```python
from build123d import *

# Parameters (mm, degrees)
SKETCH2_R          = 25
SKETCH2_R_2        = 17.5
CUT_EXTRUDE1_DEPTH = 7
SKETCH3_R          = 3
CUT_EXTRUDE2_DEPTH = 25


with BuildPart() as part:
    # Sketch1 → Revolve1 (revolve)
    with BuildSketch(Plane.XY):
        Polygon((0, 20), (0, 4), (25, 4), (25, 25), (5, 25), (5, 20), align=None)
    revolve(axis=Axis((25, 0, 0), (-1, 0, 0)))

    # Mirror1: part across plane


with BuildPart() as part_1:
    add(part.part)
    add(part.part.mirror(Plane(origin=(0, 0, 0), x_dir=(0, 0, 1), z_dir=(1, 0, 0))))

    # Sketch2 → Cut-Extrude1 (cut)
    with BuildSketch(Plane.ZY.offset(25)):
        with Locations(Location((0, 0, 0), (0, 0, 90))):
            Circle(SKETCH2_R)
        with Locations(Location((0, 0, 0), (0, 0, 270))):
            Circle(SKETCH2_R_2, mode=Mode.SUBTRACT)
    extrude(amount=-CUT_EXTRUDE1_DEPTH, mode=Mode.SUBTRACT)

    # Sketch3 → Cut-Extrude2 (cut)
    with BuildSketch(Plane(origin=(0, 25, 0), x_dir=(1, 0, 0), z_dir=(0, 1, 0))):
        with Locations(Location((-11.5, 0, 0), (0, 0, 180))):
            Circle(SKETCH3_R)
    extrude(amount=-CUT_EXTRUDE2_DEPTH, mode=Mode.SUBTRACT)


solid = part_1.part
```
CAD build for the part. Positions are in the model's coordinates, mm. A direction names the side the tool comes from. Round coordinates to 2 decimals unless told otherwise and drop trailing zeros. Loops run counter-clockwise (first coordinate to the right, second up) from the corner with the lowest first, then second, coordinate; pieces in that order, holes last. Notation, with made-up numbers: (-38, 18.5) - (-10, 18.5) arc R17 cw to (-10, 40.5) - close; hole circle Ø8 at (11.25, 74.5). An arc over 180 degrees is marked (long way). Return JSON: item names as keys, results as strings. Group by question number.
Q1. Two-plate mould, pull along X, no slides. Class faces 1 (the face through (-18, -17, 5)), 2 (the face through (-5, -11, -17)), 3 (the face through (25, 0, 5)): +X half, -X half, draft (parallel to the pull), parting line (faces both ways), or undercut.
Q2. Band-saw the part on C-C on z = 21.5. Give the cut face in (x, y), plus the area to 3 significant figures.
Q3. Tool access for faces 4 (the face through (-21.549, 13.887, -10.648)), 5 (the face through (-0.07, -4.336, 19.524)), 6 (the face through (-8.5, 14, 0.1)), 7 (the face through (-25, -4, 4)), 8 (the face through (14.86, 23.846, -7.509)): list every direction of +Z, -Z, +X, -X, +Y, -Y with a clear straight run to the whole face (end or side of a thin tool).
Q4. Band-saw the part on A-A on y = 0. Give the cut face in (x, z).
Q5. Flat gauge pins, fed straight in: pin 1 Ø3 at (x, y) = (5.5, -2.5) entering from +Z; pin 2 Ø1.5 at (x, y) = (6.5, -10.5) entering from +Z; pin 3 Ø1 at (x, z) = (-3.5, -17.5) entering from +Y. Where does each tip first touch, or does it go through?
Q6. Band-saw the part on B-B on z = 0. Give the cut face in (x, y).
Q7. Band-saw the part on D-D on x = 0.5. Give the cut face in (y, z).
Q8. Drill centre lines: line 1 along X through (y, z) = (-18.5, 11); line 2 along Y through (x, z) = (0.5, 0); line 3 along Y through (x, z) = (12, 0). Where is each one in solid material? Low to high. Write a range as [from, to].
Solutions:
{
 "1": {"face 1": "-X half", "face 2": "undercut", "face 3": "+X half"},
 "2": {"outline": "(-18, -12.76) - (-5, -12.76) - (-5, 12.76) - (-18, 12.76) - close; (5, -12.76) - (25, -12.76) - (25, 12.76) - (5, 12.76) - close", "area": "842 mm^2"},
 "3": {"face 4": "-X", "face 5": "none", "face 6": "+Y", "face 7": "+Z, -Z, -X, +Y, -Y", "face 8": "+X, -X"},
 "4": {"outline": "(-25, -17.5) - (-18, -17.5) - (-18, -25) - (-5, -25) - (-5, -20) - (5, -20) - (5, -25) - (25, -25) - (25, -4) - (-25, -4) - close; (-25, 4) - (25, 4) - (25, 25) - (5, 25) - (5, 20) - (-5, 20) - (-5, 25) - (-18, 25) - (-18, 17.5) - (-25, 17.5) - close"},
 "5": {"pin 1": "stops at z = 24.98", "pin 2": "stops at z = 23.02", "pin 3": "stops at y = 10.54"},
 "6": {"outline": "(-25, -17.5) - (-18, -17.5) - (-18, -25) - (-5, -25) - (-5, -20) - (5, -20) - (5, -25) - (25, -25) - (25, -4) - (-25, -4) - close; (-25, 4) - (-14.5, 4) - (-14.5, 25) - (-18, 25) - (-18, 17.5) - (-25, 17.5) - close; (-8.5, 4) - (25, 4) - (25, 25) - (5, 25) - (5, 20) - (-5, 20) - (-5, 25) - (-8.5, 25) - close"},
 "7": {"outline": "circle Ø40 at (0, 0); hole circle Ø8 at (0, 0)"},
 "8": {"line 1": "x = [-18, -5], [5, 25]", "line 2": "y = [-20, -4], [4, 20]", "line 3": "y = [-25, -4], [4, 25]"}
}
